Study the drawing (mm; zero at the part's minimum x, y, z) and answer. A direction names the side the tool comes from. Round coordinates to 2 decimals unless told otherwise and drop trailing zeros. Order: outer loops, then holes, each group sorted by start corner. A loop starts at its lowest first (then second) coordinate and runs counter-clockwise, first axis right, second up. Notation, with made-up numbers: (48, 20) - (90, 20) arc R9 cw to (90, 33) - close; hole circle Ø8 at (40.5, 33.5). An arc over 180 degrees is marked (long way). Put each result on its own line as item: value.
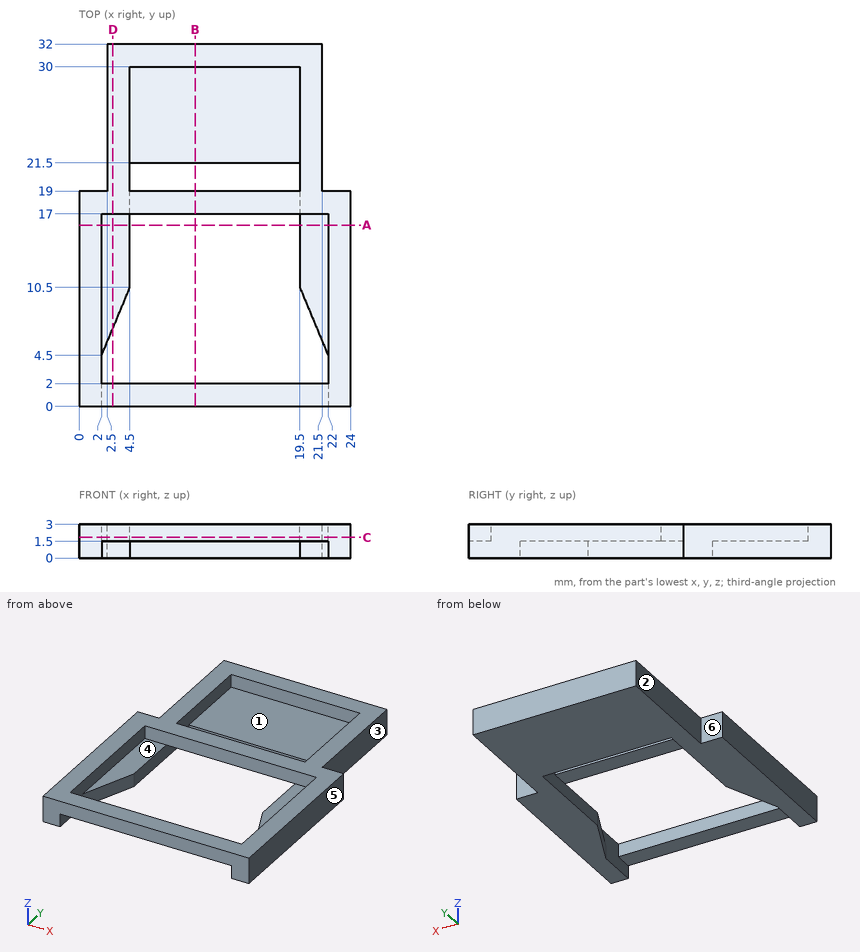
1) Straight lines are drawn through the part: L1, parallel to Y at x = 10.5, z = 2.7; L2, parallel to X at y = 22, z = 2.05; L3, parallel to X at y = 11, z = 0.25. For each, find the intervals that lie inside material, in ascending order. Write a range as from..to.
Findings below:
L1: y = 0..2, 17..19, 30..32
L2: x = 2.5..4.5, 19.5..21.5
L3: x = 0..4.5, 19.5..24
2) For the marked faces 1, 2 and 3, determine the directions among +Z, -Z, +X, -X, +Y, -Y from which every point of the face is accessible in a straight line to the end or side of a thin tool.
Findings below:
face 1: +Z
face 2: +Z, -Z, -X, +Y
face 3: +Z, -Z, +X, +Y
3) A cutting plane is placed at B-B on x = 10.25. Write down the section's boundary in (y, z).
Findings below:
outline: (0, 1.5) - (2, 1.5) - (2, 3) - (0, 3) - close; (17, 1.5) - (19, 1.5) - (19, 3) - (17, 3) - close; (21.5, 0) - (32, 0) - (32, 3) - (30, 3) - (30, 1.5) - (21.5, 1.5) - close
4) For a pull along Y with two mould halves and no side action, classify the marked faces 4, 5 and 6 as pulls with the +Y half, pulls with the -Y half, needs draft (parallel to the pull), parting line crosses it, or undercut.
Findings below:
face 4: undercut
face 5: needs draft
face 6: pulls with the +Y half
5) A cutting plane is placed at D-D on x = 3. Write down the section's boundary in (y, z).
Findings below:
outline: (0, 1.5) - (2, 1.5) - (2, 3) - (0, 3) - close; (6.9, 0) - (32, 0) - (32, 3) - (17, 3) - (17, 1.5) - (6.9, 1.5) - close
6) A cutting plane is placed at A-A on y = 16. Write down the section's boundary in (x, z).
Findings below:
outline: (0, 0) - (4.5, 0) - (4.5, 1.5) - (2, 1.5) - (2, 3) - (0, 3) - close; (19.5, 0) - (24, 0) - (24, 3) - (22, 3) - (22, 1.5) - (19.5, 1.5) - close
7) A cutting plane is placed at C-C on z = 1.85. Write down the section's boundary in (x, y).
Findings below:
outline: (0, 0) - (24, 0) - (24, 19) - (21.5, 19) - (21.5, 32) - (2.5, 32) - (2.5, 19) - (0, 19) - close; hole (2, 2) - (22, 2) - (22, 17) - (2, 17) - close; hole (4.5, 19) - (19.5, 19) - (19.5, 30) - (4.5, 30) - close
8) Given pin 1 Ø2 at (x, y) = (15.5, 1.5) entering from -Z; pin 2 Ø0.8 at (x, y) = (3.5, 7.5) entering from +Z; pin 3 Ø0.8 at (x, z) = (1, 1) entering from +Y, each flat-ended and moving along its own axis, determine where each tip first touches the part or whether it passes through.
Findings below:
pin 1: stops at z = 1.5
pin 2: stops at z = 1.5
pin 3: stops at y = 19
